Design review of the part built by this model. Coordinates are the model's own, in mm. A direction names the side the tool comes from. Round coordinates to 2 decimals unless told otherwise and drop trailing zeros. Order: outer loops, then holes, each group sorted by start corner. A loop starts at its lowest first (then second) coordinate and runs counter-clockwise, first axis right, second up. Notation, with made-up numbers: M 66.25,64 L 112.25,64 A27 cw 112.25,92 Z; hole C 32.5,11 d4. An arc over 180 degrees is marked long. Use a Markdown table: item, result. Add a question column.
(1) For pin 1 (2.5 mm diameter, centred on y = 5, z = 68, fed in from -X); pin 2 (4.5 mm diameter, centred on x = -210.5, z = 78, fed in from -Y) (3 decimals); pin 3 (1.6 mm diameter, centred on x = -210.5, y = -6, fed in from -Z), all flat-tipped, find the tip position at first contact; note any pin that passes through.
(2) The part is to be moulded in two halves that separate along X. For faces 1 (the face through (-51.18, 2.92, -7.04)), 2 (the face through (-214, 5, 70.841)), 3 (the face through (-205.102, 4, 69)), 4 (the face through (0, -8, 0)), say which applies: released by +X, released by -X, zero draft, split by the parting line, or undercut.
(3) Machinability: for faces 5 (the face through (-214, -1.905, 68)), 6 (the face through (-214, 5, 74.651)), 7 (the face through (-214, 1.905, 68)), 8 (the face through (-214, -5, 74.651)), 9 (the face through (-173.79, -0.34, 80.36)), which of the approach directions +Z, -Z, +X, -X, +Y, -Y give a long, thin tool a straight path to every point of the face, cutting with its end or side? Answer none if there is none.
(4) Take a section at A-A (x = -28). Write out the cut boundary in (y, z), then the cut area to 3 significant figures.
(5) To check wall thickness, follow probe 1 along Z at (x, y) = (-168.5, -2); probe 2 along Z at (x, y) = (-197.5, -0.5); probe 3 along Y at (x, z) = (-164, 73). State the ranges of each line that lie inside material, in increasing order. Write a range as from..to.
```python
from build123d import *

# Parameters (mm, degrees)
SKETCH3_R          = 7.62
CUT_EXTRUDE3_DEPTH = 17.78
CUT_EXTRUDE4_DEPTH = 17.78


with BuildPart() as part:
    # Sweep1: sweep along a path in Sketch1
    with BuildLine(Plane(origin=(0, 0, 0), x_dir=(1, 0, 0), z_dir=(0, 1, 0))) as sweep1_path:
        Line((0, 0), (-95.984915269, 0))
        Line((-95.984915269, 0), (-128.252610358, -72.746173646))
        Line((-128.252610358, -72.746173646), (-222.882267399, -72.746173646))
    # Sketch3 → Sweep1 (sweep)
    with BuildSketch(Plane(origin=(0, 0, 0), x_dir=(0, 0, -1), z_dir=(1, 0, 0))):
        Circle(SKETCH3_R)
    sweep(path=sweep1_path.line, transition=Transition.RIGHT)

    # Sketch6 → Revolve1 (revolve)
    with BuildSketch(Plane(origin=(0, 0, 0), x_dir=(1, 0, 0), z_dir=(0, 1, 0))):
        with BuildLine():
            Line((0, 0), (0, 11.860460566))
            ThreePointArc((0, 11.860460566), (2.307736562, 6.103805999), (3.406950908, 0))
            Line((3.406950908, 0), (0, 0))
        make_face()
    revolve(axis=Axis((0, 0, 0), (1, 0, 0)))

    # Sketch4 → Cut-Extrude3 (cut)
    with BuildSketch(Plane.ZY.offset(222.882267399)):
        with BuildLine():
            Line((80.12420692, 1.905), (74.651173646, 1.905))
            Line((74.651173646, 1.905), (74.651173646, 7.378033275))
            ThreePointArc((74.651173646, 7.378033275), (78.134327318, 5.388153673), (80.12420692, 1.905))
        make_face()
    cut_extrude3 = extrude(amount=-CUT_EXTRUDE3_DEPTH, mode=Mode.SUBTRACT)

    # Mirror3: Cut-Extrude3 across plane
    add(cut_extrude3.mirror(Plane.ZX), mode=Mode.SUBTRACT)

    # Sketch5 → Cut-Extrude4 (cut)
    with BuildSketch(Plane.ZY.offset(222.882267399)):
        with BuildLine():
            Line((65.368140371, 1.905), (70.841173646, 1.905))
            Line((70.841173646, 1.905), (70.841173646, 7.378033275))
            ThreePointArc((70.841173646, 7.378033275), (67.358019973, 5.388153673), (65.368140371, 1.905))
        make_face()
    cut_extrude4 = extrude(amount=-CUT_EXTRUDE4_DEPTH, mode=Mode.SUBTRACT)

    # Mirror4: Cut-Extrude4 across plane
    add(cut_extrude4.mirror(Plane.ZX), mode=Mode.SUBTRACT)


solid = part.part
```
Verdict:
| question | item | result |
|---|---|---|
| 1 | pin 1 | stops at x = -205.1 |
| 1 | pin 2 | stops at y = -1.905 |
| 1 | pin 3 | stops at z = 70.84 |
| 2 | face 1 | undercut |
| 2 | face 2 | zero draft |
| 2 | face 3 | released by -X |
| 2 | face 4 | undercut |
| 3 | face 5 | -Z, -X, -Y |
| 3 | face 6 | +Z, -X, +Y |
| 3 | face 7 | -Z, -X, +Y |
| 3 | face 8 | +Z, -X, -Y |
| 3 | face 9 | -X |
| 4 | outline | C 0,0 d15.24 |
| 4 | area | 182 mm^2 |
| 5 | probe 1 | z = 65.39..80.1 |
| 5 | probe 2 | z = 65.14..80.35 |
| 5 | probe 3 | y = -7.62..7.62 |
